Geometry check sheet. Reference: the model listing, model coordinates, mm. A direction names the side the tool comes from. Coordinates: 2 decimals unless noted, no trailing zeros. Write each loop counter-clockwise with the first axis right and the second up, starting at its lowest first coordinate (ties: lowest second). Pieces come first, ordered by that corner, then holes. Notation, with made-up numbers: (61.5, 74) -> (86.5, 74) arc R7 cw to (86.5, 85) -> close; hole circle Ø10 at (74, -28.75). An arc over 180 degrees is marked (long way). Use a Markdown table: item, result.
```python
from build123d import *

# Parameters (mm, degrees)
CROQUIS1_W              = 200
CROQUIS1_H              = 200
SALIENTE_EXTRUIR1_DEPTH = 10
CROQUIS2_W              = 20
CROQUIS2_H              = 20
CROQUIS2_H_2            = 15
CROQUIS2_W_2            = 15
CORTAR_EXTRUIR1_DEPTH   = 3
CORTAR_EXTRUIR2_DEPTH   = 10
CROQUIS4_R              = 5
CORTAR_EXTRUIR3_DEPTH   = 10


with BuildPart() as part:
    # Croquis1 → Saliente-Extruir1 (new body)
    with BuildSketch(Plane(origin=(0, 0, 0), x_dir=(1, 0, 0), z_dir=(0, 1, 0))):
        Rectangle(CROQUIS1_W, CROQUIS1_H)
    extrude(amount=SALIENTE_EXTRUIR1_DEPTH)

    # Croquis2 → Cortar-Extruir1 (cut)
    with BuildSketch(Plane(origin=(0, 10, 0), x_dir=(1, 0, 0), z_dir=(0, 1, 0))):
        Rectangle(CROQUIS2_W, CROQUIS2_H)
        with Locations((0, 52.5)):
            Rectangle(CROQUIS2_W, CROQUIS2_H_2)
        with Locations((52.5, 0)):
            Rectangle(CROQUIS2_W_2, CROQUIS2_H)
    extrude(amount=-CORTAR_EXTRUIR1_DEPTH, mode=Mode.SUBTRACT)

    # Croquis3 → Cortar-Extruir2 (cut)
    with BuildSketch(Plane(origin=(0, 10, 0), x_dir=(1, 0, 0), z_dir=(0, 1, 0))):
        with BuildLine():
            Line((100, 100), (20, 100))
            ThreePointArc((20, 100), (43.431457505, 43.431457505), (100, 20))
            Line((100, 20), (100, 100))
        make_face()
        with BuildLine():
            ThreePointArc((-100, 20), (-43.431457505, 43.431457505), (-20, 100))
            Line((-20, 100), (-100, 100))
            Line((-100, 100), (-100, 20))
        make_face()
        with BuildLine():
            ThreePointArc((-20, -100), (-43.431457505, -43.431457505), (-100, -20))
            Line((-100, -20), (-100, -100))
            Line((-100, -100), (-20, -100))
        make_face()
        with BuildLine():
            Line((100, -100), (100, -20))
            ThreePointArc((100, -20), (43.431457505, -43.431457505), (20, -100))
            Line((20, -100), (100, -100))
        make_face()
    extrude(amount=-CORTAR_EXTRUIR2_DEPTH, mode=Mode.SUBTRACT)

    # Croquis4 → Cortar-Extruir3 (cut)
    with BuildSketch(Plane(origin=(0, 10, 0), x_dir=(1, 0, 0), z_dir=(0, 1, 0))):
        with Locations(Location((-78.897440542, 0, 0), (0, 0, 270))):
            Circle(CROQUIS4_R)
        with Locations(Location((1.102559458, 80, 0), (0, 0, 270))):
            Circle(CROQUIS4_R)
        with Locations(Location((81.102559458, 0, 0), (0, 0, 270))):
            Circle(CROQUIS4_R)
        with Locations(Location((1.102559458, -80, 0), (0, 0, 270))):
            Circle(CROQUIS4_R)
    extrude(amount=-CORTAR_EXTRUIR3_DEPTH, mode=Mode.SUBTRACT)


solid = part.part
```
Item 1: Depth check by flat-ended pin: P1, Ø1, axis at y = 3, z = -30.5, coming from the -X side; P2, Ø1, axis at x = 40, y = 4, coming from the +Z side; P3, Ø3.5, axis at x = 51, y = 8, coming from the -Z side; P4, Ø9, axis at x = -78.9, z = 0, coming from the +Y side. Enter the tip coordinate at first touch or a pass-through.
Answer block:
| item | result |
|---|---|
| P1 | stops at x = -61.27 |
| P2 | stops at z = 47.66 |
| P3 | stops at z = -38.16 |
| P4 | passes through |
Item 2: Section check B-B on z = -80. Record the boundary of the cut face in (x, y).
Answer block:
| item | result |
|---|---|
| outline | (-22.54, 0) -> (-3.9, 0) -> (-3.9, 10) -> (-22.54, 10) -> close; (6.1, 0) -> (22.54, 0) -> (22.54, 10) -> (6.1, 10) -> close |
Item 3: Section check C-C on y = 2.5. Record the boundary of the cut face in (x, z).
Answer block:
| item | result |
|---|---|
| outline | (-100, -20) arc R80 cw to (-20, -100) -> (20, -100) arc R80 cw to (100, -20) -> (100, 20) arc R80 cw to (20, 100) -> (-20, 100) arc R80 cw to (-100, 20) -> close; hole circle Ø10 at (-78.9, 0); hole circle Ø10 at (1.1, -80); hole circle Ø10 at (1.1, 80); hole circle Ø10 at (81.1, 0) |
Item 4: Tool access check on faces 4 (the flat face through (0, 7, -53)), 5 (the flat face through (0, 5, -100)). Record the directions out of +Z, -Z, +X, -X, +Y, -Y that give a thin tool (end or side, any length) a straight path to the whole face; none if there is none.
Answer block:
| item | result |
|---|---|
| face 4 | +Y |
| face 5 | -Z, +X, -X, +Y, -Y |
Item 5: Section check A-A on z = 0. Record the boundary of the cut face in (x, y), then the cut area to 4 significant figures.
Answer block:
| item | result |
|---|---|
| outline | (-100, 0) -> (-83.9, 0) -> (-83.9, 10) -> (-100, 10) -> close; (-73.9, 0) -> (76.1, 0) -> (76.1, 10) -> (60, 10) -> (60, 7) -> (45, 7) -> (45, 10) -> (10, 10) -> (10, 7) -> (-10, 7) -> (-10, 10) -> (-73.9, 10) -> close; (86.1, 0) -> (100, 0) -> (100, 10) -> (86.1, 10) -> close |
| area | 1,695 mm^2 |
Item 6: Thickness scan on L1, parallel to X at y = 5.75, z = 0; L2, parallel to Z at x = -5, y = 8.25; L3, parallel to Z at x = -3.5, y = 9. Record the ranges inside material, lowest first. Write a range as [from, to].
Answer block:
| item | result |
|---|---|
| L1 | x = [-100, -83.9], [-73.9, 76.1], [86.1, 100] |
| L2 | z = [-100, -60], [-45, -10], [10, 100] |
| L3 | z = [-100, -81.95], [-78.05, -60], [-45, -10], [10, 78.05], [81.95, 100] |
Item 7: Mould release check, pull along Z, two halves, no side actions. Record for faces 1 (the cylindrical face through (-44.06, 5.07, -42.81)), 2 (the flat face through (-1, 10, 21)), 3 (the cylindrical face through (-0.81, 5.07, -75.38)): +Z half, -Z half, draft (parallel to the pull), parting line (faces both ways), or undercut.
Answer block:
| item | result |
|---|---|
| face 1 | -Z half |
| face 2 | draft |
| face 3 | undercut |
Item 8: Section check D-D on x = 22.5. Record the boundary of the cut face in (y, z).
Answer block:
| item | result |
|---|---|
| outline | (0, -80.16) -> (10, -80.16) -> (10, 80.16) -> (0, 80.16) -> close |
